from build123d import *

# Parameters (mm, degrees)
BOSS_EXTRUDE1_DEPTH = 4
SKETCH2_R           = 1.5
BOSS_EXTRUDE2_DEPTH = 37
SKETCH3_R           = 2.086060033
BOSS_EXTRUDE3_DEPTH = 2
SKETCH4_W           = 5
SKETCH4_H           = 3.576334768
CUT_EXTRUDE1_DEPTH  = 32
SKETCH5_R           = 2
BOSS_EXTRUDE4_DEPTH = 12


with BuildPart() as part:
    # Sketch1 → Boss-Extrude1 (new body)
    with BuildSketch(Plane(origin=(0, 0, 0), x_dir=(1, 0, 0), z_dir=(0, 1, 0))):
        with BuildLine():
            Line((-2, 0), (-2, 20))
            ThreePointArc((-2, 20), (0, 22), (2, 20))
            Line((2, 20), (2, 0))
            ThreePointArc((2, 0), (0, -2), (-2, 0))
        make_face()
    extrude(amount=BOSS_EXTRUDE1_DEPTH)

    # Sketch2 → Boss-Extrude2 (add)
    with BuildSketch(Plane(origin=(0, 12, 0), x_dir=(1, 0, 0), z_dir=(0, 1, 0))):
        Circle(SKETCH2_R)
    extrude(amount=-BOSS_EXTRUDE2_DEPTH)

    # Sketch3 → Boss-Extrude3 (add)
    with BuildSketch(Plane.XZ.offset(25)):
        Circle(SKETCH3_R)
    extrude(amount=BOSS_EXTRUDE3_DEPTH)

    # Sketch4 → Cut-Extrude1 (cut, through all)
    with BuildSketch(Plane(origin=(0, 4, 0), x_dir=(1, 0, 0), z_dir=(0, 1, 0))):
        with Locations((0.5, 21.788167384)):
            Rectangle(SKETCH4_W, SKETCH4_H)
    extrude(amount=-CUT_EXTRUDE1_DEPTH, mode=Mode.SUBTRACT)

    # Sketch5 → Boss-Extrude4 (add)
    with BuildSketch(Plane(origin=(0, 0, -20), x_dir=(-1, 0, 0), z_dir=(0, 0, -1))):
        with Locations((0, 2)):
            Circle(SKETCH5_R)
    extrude(amount=BOSS_EXTRUDE4_DEPTH)


solid = part.part
Geometry check sheet. Reference: the model listing, model coordinates, mm. A direction names the side the tool comes from. Coordinates: 2 decimals unless noted, no trailing zeros. Order: outer loops, then holes, each group sorted by start corner. A loop starts at its lowest first (then second) coordinate and runs counter-clockwise, first axis right, second up. Notation, with made-up numbers: (53, 49.25) - (68, 49.25) arc R19 ccw to (68, 73.25) - close; hole circle Ø10 at (-28.75, 20). An arc over 180 degrees is marked (long way). Answer in a Markdown table with one row per item. Add a question column.
1) Material ranges on line 1 along Y through (x, z) = (-1.5, -19.5); line 2 along X through (y, z) = (2, -3.5); line 3 along Z through (x, y) = (-0.1, -9), recorded low to high. Write a range as [from, to].
2) Cross-section at C-C, the plane y = -10.5. Record the cut outline in (x, z), then the cut area to 3 significant figures.
3) Cross-section at B-B, the plane y = 3. Record the cut outline in (x, z).
4) Release check for a two-part mould opening along Y. For faces 4 (the flat face through (0, 2, -32)), 5 (the flat face through (0, 4, -9)), 6 (the flat face through (0.9, -25, -1.4)) record: +Y half, -Y half, draft (parallel to the pull), parting line (faces both ways), or undercut.
5) Set-up check for faces 1 (the cylindrical face through (-1.5, 8.06, -0.07)), 2 (the cylindrical face through (0, 0, -26)), 3 (the flat face through (-1.6, 3.5, -20)): record each of +Z, -Z, +X, -X, +Y, -Y from which the full face is reachable in a straight line by a thin tool's end or side.
6) Cross-section at A-A, the plane z = -26.5. Record the cut outline in (x, y).
7) Cross-section at D-D, the plane z = -15.5. Record the cut outline in (x, y), then the cut area to 3 significant figures.
8) Gauge pin test, flat ends, axial feed: P1, Ø1.2, axis at x = -0.5, z = -10.5, coming from the -Y side; P2, Ø2, axis at x = 1, z = -14, coming from the +Y side; P3, Ø2, axis at y = -11.5, z = -3.5, coming from the +X side; P4, Ø4.5, axis at y = 1, z = -10.5, coming from the +X side. Record the tip position at first contact, or that the pin passes through.
Check result:
| question | item | result |
|---|---|---|
| 1 | line 1 | y = [0, 4] |
| 1 | line 2 | x = [-2, 2] |
| 1 | line 3 | z = [-1.5, 1.5] |
| 2 | outline | circle Ø3 at (0, 0) |
| 2 | area | 7.07 mm² |
| 3 | outline | (-2, -20) - (-1.73, -20) - (-1.73, -32) - (1.73, -32) - (1.73, -20) - (2, -20) - (2, 0) arc R2 ccw to (-2, 0) - close |
| 4 | face 4 | draft |
| 4 | face 5 | +Y half |
| 4 | face 6 | undercut |
| 5 | face 1 | +Y |
| 5 | face 2 | -Z |
| 5 | face 3 | -Z, -X, +Y |
| 6 | outline | circle Ø4 at (0, 2) |
| 7 | outline | (-2, 0) - (2, 0) - (2, 4) - (-2, 4) - close |
| 7 | area | 16.0 mm² |
| 8 | P1 | stops at y = 0 |
| 8 | P2 | stops at y = 4 |
| 8 | P3 | passes through |
| 8 | P4 | stops at x = 2 |
